The model under review builds one solid part; all positions refer to its coordinate system, in mm. Coordinates: 2 decimals unless noted, no trailing zeros. Order: outer loops, then holes, each group sorted by start corner. A loop starts at its lowest first (then second) coordinate and runs counter-clockwise, first axis right, second up. Notation, with made-up numbers: M 79.25,-26 L 88.25,-26 A8 ccw 88.25,-14 Z; hole C 67,71 d9. An arc over 180 degrees is marked long. Answer as CSV lines item,"result". Start each with the question number.
Q1. Wall thickness on L1, parallel to X at y = 1.5, z = -1; L2, parallel to X at y = 2.25, z = 0; L3, parallel to X at y = 1.75, z = -2.25: over which ranges is each line inside the solid? List them lowest first. Write a range as [from, to].
Q2. Consider section B-B on x = 4.75. Write out the cut boundary in (y, z).
Q3. The part is to be moulded in two halves that separate along Y. For faces 1 (the face through (10.75, -1.33, -0.17)), 2 (the face through (4, 2, 2)), 3 (the face through (1.183, 0.905, 0.513)), say which applies: +Y half, -Y half, draft (parallel to the pull), parting line (faces both ways), or undercut.
Q4. For P1, Ø5, axis at x = 10.5, z = -0.5, coming from the -Y side; P2, Ø1, axis at x = 9.5, y = 2, coming from the +Z side; P3, Ø5, axis at x = 9, z = -3.5, coming from the +Y side, all flat-tipped, find the tip position at first contact; note any pin that passes through.
Q5. Consider section A-A on x = 1. Write out the cut boundary in (y, z), and give its area (3 significant figures).
from build123d import *

# Parameters (mm, degrees)
CHAMFER1_SIZE   = 0.01
HEX_2_DEPTH     = 2.4
THDSCHPAT_COUNT = 4
THDSCHPAT_PITCH = 0.8


with BuildPart() as part:
    # BodySke → BaseBody (revolve)
    with BuildSketch(Plane.XY, mode=Mode.PRIVATE) as basebody_sk:
        with BuildLine():
            Line((0, 0), (0, 4.5))
            Line((0, 4.5), (4, 4.5))
            Line((4, 4.5), (4, 2.36))
            ThreePointArc((4, 2.36), (4.002928932, 2.352928932), (4.01, 2.35))
            Line((4.01, 2.35), (4.45, 2.35))
            Line((4.45, 2.35), (4.5, 2.4))
            Line((4.5, 2.4), (10, 2.4))
            Line((10, 2.4), (10, 1.84))
            ThreePointArc((10, 1.84), (10.146446609, 1.486446609), (10.5, 1.34))
            Line((10.5, 1.34), (11, 1.34))
            Line((11, 1.34), (11.66, 2))
            Line((11.66, 2), (14.61, 2))
            Line((14.61, 2), (15, 1.61))
            Line((15, 1.61), (15, 0))
            Line((15, 0), (0, 0))
        make_face()
    revolve(basebody_sk.sketch.rotate(Axis((-6.35, 0, 0), (1, 0, 0)), 90), axis=Axis((-6.35, 0, 0), (1, 0, 0)))

    # Chamfer1
    chamfer1_edges = [part.edges().sort_by_distance(p)[0] for p in [
        (0, 0, -4.5),
    ]]
    chamfer(chamfer1_edges, length=CHAMFER1_SIZE)

    # Sketch2 → PreBroach (revolve, cut)
    with BuildSketch(Plane.XY, mode=Mode.PRIVATE) as prebroach_sk:
        Polygon((0, 1.04), (2, 1.04), (2.60044428, 0), (0, 0), align=None)
    revolve(prebroach_sk.sketch.rotate(Axis((0, 0, 0), (1, 0, 0)), 90), axis=Axis((0, 0, 0), (1, 0, 0)), mode=Mode.SUBTRACT)

    # Sketch3 → Hex 2 (cut)
    with BuildSketch(Plane.ZY):
        Polygon((-1.04, -0.60044428), (-1.04, 0.60044428), (0, 1.20088856), (1.04, 0.60044428), (1.04, -0.60044428), (0, -1.20088856), align=None)
    extrude(amount=-HEX_2_DEPTH, mode=Mode.SUBTRACT)

    # ThdSchSke → ThreadSchematic (revolve, cut)
    with BuildSketch(Plane.XY):
        Polygon((11.8, -1.61), (11.246836045, -2.4), (11.246836045, -3), (12.353163955, -3), (12.353163955, -2.4), align=None)
    threadschematic = revolve(axis=Axis((-3.175, 0, 0), (1, 0, 0)), mode=Mode.SUBTRACT)

    # ThdSchPat: ThreadSchematic ×4
    with Locations(*[(i * THDSCHPAT_PITCH, 0, 0) for i in range(1, THDSCHPAT_COUNT)]):
        add(threadschematic, mode=Mode.SUBTRACT)


solid = part.part
Evaluation:
1,L1,"x = [0, 10], [11.46, 11.67], [11.93, 12.47], [12.73, 13.27], [13.53, 14.07], [14.33, 14.81]"
1,L2,"x = [0, 10]"
1,L3,"x = [0, 4]"
2,outline,"C 0,0 d4.8"
3,face 1,"parting line"
3,face 2,"draft"
3,face 3,"undercut"
4,P1,"stops at y = -2.4"
4,P2,"stops at z = 1.87"
4,P3,"stops at y = 2.18"
5,outline,"C 0,0 d9; hole M -1.2,0 L -0.6,-1.04 L 0.6,-1.04 L 1.2,0 L 0.6,1.04 L -0.6,1.04 Z"
5,area,"59.9 mm²"
